Verification items for this drawing (mm, ordinates from the low corner). Round coordinates to 2 decimals unless told otherwise and drop trailing zeros. Loops run counter-clockwise (first coordinate to the right, second up) from the corner with the lowest first, then second, coordinate; pieces in that order, holes last. Notation, with made-up numbers: (73, 28) - (129, 28) arc R8 ccw to (129, 35) - close; hole circle Ø2 at (43, 40). An arc over 180 degrees is marked (long way). Put each result on its own line as item: value. Start each with the question number.
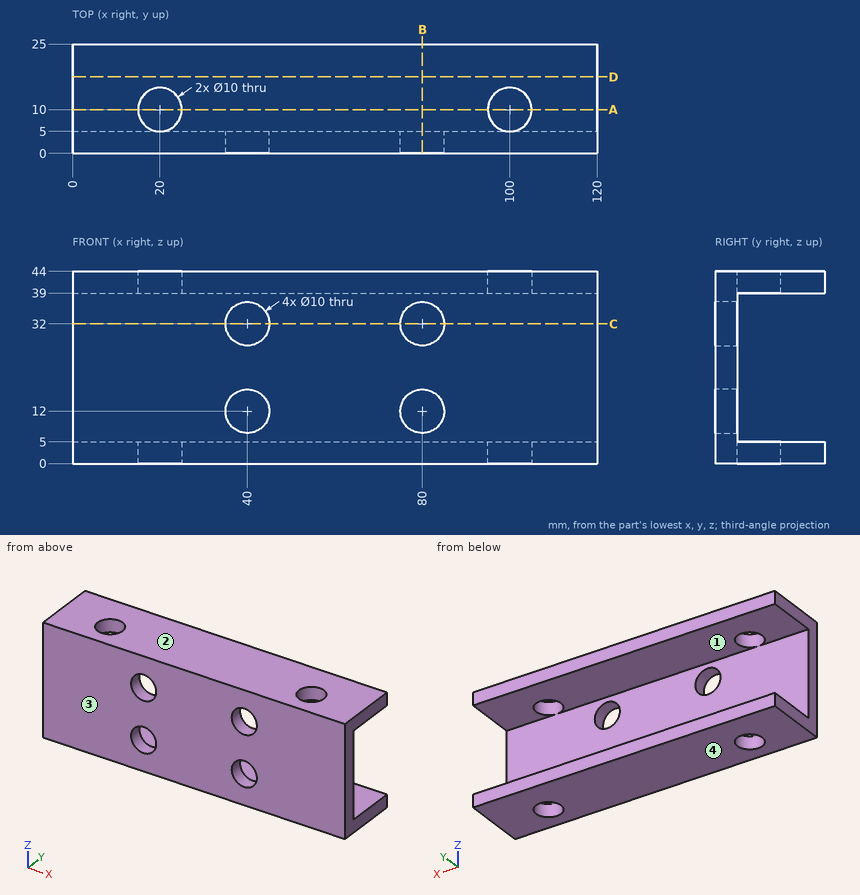
Q1. Material ranges on line 1 (X direction, y = 10, z = 3.65); line 2 (X direction, y = 3.9, z = 32); line 3 (Z direction, x = 57.5, y = 15.5), recorded low to high. Write a range as from..to.
Q2. Cross-section at A-A on y = 10. Enter the section's corners in (x, z), and give its area (3 significant figures).
Q3. Cross-section at C-C on z = 32. Enter the section's corners in (x, y).
Q4. Draft check along Z on the marked faces 1, 2, 3 and 4. Enter one of: +Z half, -Z half, draft (parallel to the pull), parting line (faces both ways), or undercut.
Q5. Cross-section at B-B on x = 80. Enter the section's corners in (y, z), and give its area (3 significant figures).
Q6. Cross-section at D-D on y = 17.5. Enter the section's corners in (x, z), and give its area (3 significant figures).
Q7. Depth check by flat-ended pin: pin 1 Ø13 at (x, y) = (20, 10) entering from +Z; pin 2 Ø11.5 at (x, z) = (80, 32) entering from +Y; pin 3 Ø9 at (x, y) = (20, 10) entering from +Z. Enter the tip coordinate at first touch or a pass-through.
Answer list:
1. line 1: x = 0..15, 25..95, 105..120
1. line 2: x = 0..35, 45..75, 85..120
1. line 3: z = 0..5, 39..44
2. outline: (0, 0) - (15, 0) - (15, 5) - (0, 5) - close; (0, 39) - (15, 39) - (15, 44) - (0, 44) - close; (25, 0) - (95, 0) - (95, 5) - (25, 5) - close; (25, 39) - (95, 39) - (95, 44) - (25, 44) - close; (105, 0) - (120, 0) - (120, 5) - (105, 5) - close; (105, 39) - (120, 39) - (120, 44) - (105, 44) - close
2. area: 1,000 mm2
3. outline: (0, 0) - (35, 0) - (35, 5) - (0, 5) - close; (45, 0) - (75, 0) - (75, 5) - (45, 5) - close; (85, 0) - (120, 0) - (120, 5) - (85, 5) - close
4. face 1: undercut
4. face 2: +Z half
4. face 3: draft
4. face 4: -Z half
5. outline: (0, 0) - (25, 0) - (25, 5) - (5, 5) - (5, 7) - (0, 7) - close; (0, 17) - (5, 17) - (5, 27) - (0, 27) - close; (0, 37) - (5, 37) - (5, 39) - (25, 39) - (25, 44) - (0, 44) - close
5. area: 320 mm2
6. outline: (0, 0) - (120, 0) - (120, 5) - (0, 5) - close; (0, 39) - (120, 39) - (120, 44) - (0, 44) - close
6. area: 1,200 mm2
7. pin 1: stops at z = 44
7. pin 2: stops at y = 5
7. pin 3: passes through
